from build123d import *

# Parameters (mm, degrees)
SKETCH1_R           = 2.999994
BOSS_EXTRUDE1_DEPTH = 6.858
SKETCH2_W           = 50.8
SKETCH2_H           = 9.525
BOSS_EXTRUDE2_DEPTH = 24.892
CUT_EXTRUDE1_DEPTH  = 24.892
SKETCH4_W           = 6.35
SKETCH4_H           = 18.373928642
CUT_EXTRUDE2_DEPTH  = 58.166


with BuildPart() as part:
    # Sketch1 → Boss-Extrude1 (new body)
    with BuildSketch(Plane(origin=(0, 0, 0), x_dir=(1, 0, 0), z_dir=(0, 1, 0))):
        with BuildLine():
            Line((22.86, -25.4), (-22.86, -25.4))
            ThreePointArc((-22.86, -25.4), (-24.656051224, -24.656051224), (-25.4, -22.86))
            Line((-25.4, -22.86), (-25.4, 22.86))
            ThreePointArc((-25.4, 22.86), (-24.656051224, 24.656051224), (-22.86, 25.4))
            Line((-22.86, 25.4), (22.86, 25.4))
            ThreePointArc((22.86, 25.4), (24.656051224, 24.656051224), (25.4, 22.86))
            Line((25.4, 22.86), (25.4, -22.86))
            ThreePointArc((25.4, -22.86), (24.656051224, -24.656051224), (22.86, -25.4))
        make_face()
        with Locations(Location((-18.499963, 18.499963, 0), (0, 0, 270))):
            Circle(SKETCH1_R, mode=Mode.SUBTRACT)
        with Locations(Location((18.499963, 18.499963, 0), (0, 0, 270))):
            Circle(SKETCH1_R, mode=Mode.SUBTRACT)
        with Locations(Location((18.499963, -18.499963, 0), (0, 0, 270))):
            Circle(SKETCH1_R, mode=Mode.SUBTRACT)
        with Locations(Location((-18.499963, -18.499963, 0), (0, 0, 270))):
            Circle(SKETCH1_R, mode=Mode.SUBTRACT)
    extrude(amount=BOSS_EXTRUDE1_DEPTH)

    # Sketch2 → Boss-Extrude2 (add)
    with BuildSketch(Plane(origin=(0, 6.858, 0), x_dir=(1, 0, 0), z_dir=(0, 1, 0))):
        with Locations((0, -4.7625)):
            Rectangle(SKETCH2_W, SKETCH2_H)
        with Locations((0, 4.7625)):
            Rectangle(SKETCH2_W, SKETCH2_H)
    extrude(amount=BOSS_EXTRUDE2_DEPTH)

    # Sketch3 → Cut-Extrude1 (cut)
    with BuildSketch(Plane.XY.offset(9.525)):
        with BuildLine():
            ThreePointArc((6.35, 16.103217479), (4.490128061, 20.593345539), (0, 22.453217479))
            Line((0, 22.453217479), (0, 9.753217479))
            ThreePointArc((0, 9.753217479), (4.490128061, 11.613089418), (6.35, 16.103217479))
        make_face()
        with BuildLine():
            Line((0, 9.753217479), (0, 22.453217479))
            ThreePointArc((0, 22.453217479), (-6.35, 16.103217479), (0, 9.753217479))
        make_face()
        with BuildLine():
            Line((25.4, 31.75), (0, 31.75))
            Line((0, 31.75), (0, 25.231928642))
            ThreePointArc((0, 25.231928642), (15.674511585, 20.156909879), (25.4, 6.858))
            Line((25.4, 6.858), (25.4, 31.75))
        make_face()
        with BuildLine():
            Line((0, 25.231928642), (0, 31.75))
            Line((0, 31.75), (-25.4, 31.75))
            Line((-25.4, 31.75), (-25.4, 6.858))
            ThreePointArc((-25.4, 6.858), (-15.674511585, 20.156909879), (0, 25.231928642))
        make_face()
    extrude(amount=-CUT_EXTRUDE1_DEPTH, mode=Mode.SUBTRACT)

    # Sketch4 → Cut-Extrude2 (cut)
    with BuildSketch(Plane.ZY.offset(25.4)):
        Polygon((-9.525, 25.231928642), (-9.525, 6.858), (-3.175, 6.858), (-3.175, 25.231928642), (-5.096857021, 25.231928642), align=None)
        with Locations((6.35, 16.044964321)):
            Rectangle(SKETCH4_W, SKETCH4_H)
    extrude(amount=-CUT_EXTRUDE2_DEPTH, mode=Mode.SUBTRACT)


solid = part.part
Can you work these out from the model? Positions are in its coordinate system, mm. A direction names the side the tool comes from. Round coordinates to 2 decimals unless told otherwise and drop trailing zeros. Write each loop counter-clockwise with the first axis right and the second up, starting at its lowest first coordinate (ties: lowest second). Pieces come first, ordered by that corner, then holes. Notation, with made-up numbers: (29.25, 52.5) -> (71.25, 52.5) arc R24 cw to (71.25, 77.5) -> close; hole circle Ø1 at (77, 44). An arc over 180 degrees is marked (long way). One line per question, with ' | ' between items. Start each with the question number.
1) I need wall thicknesses on line 1 (X direction, y = 4.75, z = -20); line 2 (Y direction, x = -21.5, z = -5); line 3 (Z direction, x = -12, y = 14.5) (3 decimals). Which ranges of each line are inside material? Lowest first, please. Write a range as [from, to].
2) I'm going to push flat-ended pins straight in: P1, Ø9.5, axis at x = 18.5, z = -18.5, coming from the +Y side; P2, Ø8, axis at y = 18.5, z = 1.5, coming from the +X side; P3, Ø2, axis at y = 22, z = -3.5, coming from the -X side. Where does each tip first touch, or does it pass through?
3) Suppose I cut it at D-D on y = 17.5. Write out the boundary of the cut face in (x, z) (3 decimals), then the cut area to 3 significant figures.
4) Suppose I cut it at A-A on y = 10.5. Write out the boundary of the cut face in (x, z) (3 decimals).
5) If we mould it in two halves opening along Z, with no side actions, what happens to faces 4 (the flat face through (0, 3, -25.4)), 5 (the cylindrical face through (15.57, 3.38, -19.15)), 6 (the flat face through (0, 0, 0))? For each: released by +Z, released by -Z, zero draft, split by the parting line, or undercut.
6) Suppose I cut it at B-B on y = 3.5. Write out the boundary of the cut face in (x, z).
7) On a 3-axis mill with a long thin cutter (end or side, diameter ignored), from which of +Z, -Z, +X, -X, +Y, -Y can I reach the whole of each face in a straight line? I mean faces 1 (the flat face through (0, 6.858, 14)), 2 (the flat face through (0, 3, 25.4)), 3 (the flat face through (-6, 12, -3.175)). Say none if no direction works.
8) Suppose I cut it at C-C on z = 17.5. Write out the boundary of the cut face in (x, y).
Return value:
1) line 1: x = [-25.4, -21.1], [-15.9, 15.9], [21.1, 25.4] | line 2: y = [0, 6.86] | line 3: z = [-3.175, 3.175]
2) P1: stops at y = 6.86 | P2: stops at x = 21.42 | P3: stops at x = -14.35
3) outline: (-18.809, -3.175) -> (-6.194, -3.175) -> (-6.194, 3.175) -> (-18.809, 3.175) -> close; (6.194, -3.175) -> (18.809, -3.175) -> (18.809, 3.175) -> (6.194, 3.175) -> close | area: 160 mm2
4) outline: (-23.894, -3.175) -> (-2.988, -3.175) -> (-2.988, 3.175) -> (-23.894, 3.175) -> close; (2.988, -3.175) -> (23.894, -3.175) -> (23.894, 3.175) -> (2.988, 3.175) -> close
5) face 4: released by -Z | face 5: undercut | face 6: zero draft
6) outline: (-25.4, -22.86) arc R2.54 ccw to (-22.86, -25.4) -> (22.86, -25.4) arc R2.54 ccw to (25.4, -22.86) -> (25.4, 22.86) arc R2.54 ccw to (22.86, 25.4) -> (-22.86, 25.4) arc R2.54 ccw to (-25.4, 22.86) -> close; hole circle Ø6 at (-18.5, -18.5); hole circle Ø6 at (-18.5, 18.5); hole circle Ø6 at (18.5, -18.5); hole circle Ø6 at (18.5, 18.5)
7) face 1: +Z, +X, -X, +Y | face 2: +Z, +X, -X, +Y, -Y | face 3: -Z, +X, -X, +Y
8) outline: (-25.4, 0) -> (-21.33, 0) -> (-21.33, 6.86) -> (-25.4, 6.86) -> close; (-15.67, 0) -> (15.67, 0) -> (15.67, 6.86) -> (-15.67, 6.86) -> close; (21.33, 0) -> (25.4, 0) -> (25.4, 6.86) -> (21.33, 6.86) -> close
